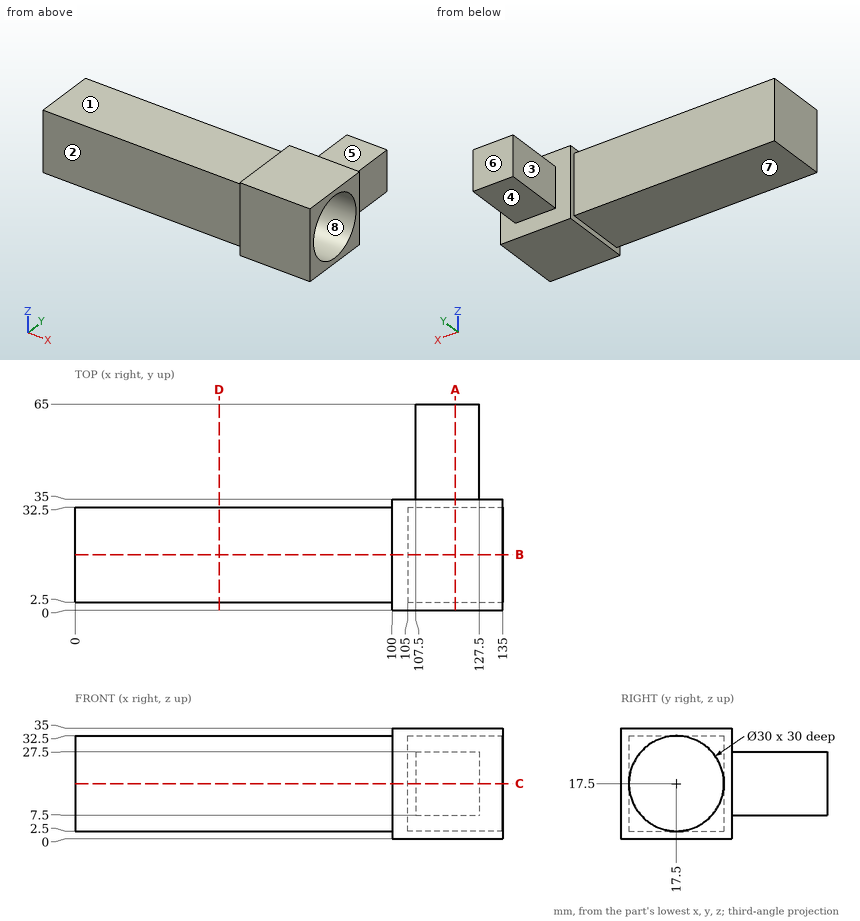
Can you work these out from the drawing? Everything is in mm from the part's minimum corner. A direction names the side the tool comes from. Coordinates: 2 decimals unless noted, no trailing zeros. Loops run counter-clockwise (first coordinate to the right, second up) from the corner with the lowest first, then second, coordinate; pieces in that order, holes last. Notation, with made-up numbers: (-21, -29) - (-14, -29) arc R23 ccw to (-14, -13) - close; hole circle Ø6 at (14.25, 88.25). An arc over 180 degrees is marked (long way). Put each result on its own line as item: value. Start each with the question number.
Item 1: Suppose I cut it at C-C (z = 17.5). Please give me the cut outline in (x, y).
Item 2: If we mould it in two halves opening along Z, with no side actions, what happens to the marked faces 6, 7 and 8? For each: +Z half, -Z half, draft (parallel to the pull), parting line (faces both ways), or undercut.
Item 3: If I drill on line 1 along Y through (x, z) = (113, 17); line 2 along Z through (x, y) = (126, 17); line 3 along Z through (x, y) = (82, 7.5), over which ranges is the centre line in solid material (lowest first)?
Item 4: For pin 1 (15 mm diameter, centred on x = 37, y = 14, fed in from -Z); pin 2 (18 mm diameter, centred on y = 17.5, z = 17.5, fed in from +X); pin 3 (16 mm diameter, centred on y = 52.5, z = 15, fed in from -X), each with a flat end and sliding along its axis, tell me the tip position at first contact or that it passes through.
Item 5: Suppose I cut it at B-B (y = 17.5). Please give me the cut outline in (x, z), and give its area (4 significant figures).
Item 6: Suppose I cut it at D-D (x = 45.5). Please give me the cut outline in (y, z).
Item 7: Which directions (+Z, -Z, +X, -X, +Y, -Y) give clear straight access to the entire face, cutting with the end or side of a thin tool? Please do the marked faces 1, 2, 3, 4 and 5.
Item 8: Suppose I cut it at A-A (x = 120). Please give me the cut outline in (y, z), and give its area (3 significant figures).
Here are the results:
1. outline: (0, 2.5) - (100, 2.5) - (100, 0) - (135, 0) - (135, 2.5) - (105, 2.5) - (105, 32.5) - (135, 32.5) - (135, 35) - (127.5, 35) - (127.5, 65) - (107.5, 65) - (107.5, 35) - (100, 35) - (100, 32.5) - (0, 32.5) - close
2. face 6: draft
2. face 7: -Z half
2. face 8: undercut
3. line 1: 0 to 2.51, 32.49 to 65
3. line 2: 0 to 2.51, 32.49 to 35
3. line 3: 2.5 to 32.5
4. pin 1: z = 2.5
4. pin 2: x = 105
4. pin 3: x = 107.5
5. outline: (0, 2.5) - (100, 2.5) - (100, 0) - (135, 0) - (135, 2.5) - (105, 2.5) - (105, 32.5) - (135, 32.5) - (135, 35) - (100, 35) - (100, 32.5) - (0, 32.5) - close
5. area: 3,325 mm²
6. outline: (2.5, 2.5) - (32.5, 2.5) - (32.5, 32.5) - (2.5, 32.5) - close
7. face 1: +Z, -X, +Y, -Y
7. face 2: +Z, -Z, -X, -Y
7. face 3: +Z, -Z, -X, +Y
7. face 4: -Z, +X, -X, +Y
7. face 5: +Z, +X, -X, +Y
8. outline: (0, 0) - (35, 0) - (35, 7.5) - (65, 7.5) - (65, 27.5) - (35, 27.5) - (35, 35) - (0, 35) - close; hole circle Ø30 at (17.5, 17.5)
8. area: 1,120 mm²
